from build123d import *

# Parameters (mm, degrees)
F1_DEPTH = 25.4
F2_W     = 25.4
F2_H     = 12.7
F3_DEPTH = 25.4
F4_R     = 6.35
F5_DEPTH = 76.201
F6_R     = 12.7


with BuildPart() as f1:
    # F0 (on Front) → F1 (new body, symmetric)
    with BuildSketch(Plane.XZ):
        Polygon((0, 38.1), (0, 0), (76.2, 0), (76.2, 12.7), (50.8, 12.7), (50.8, 25.4), (25.4, 25.4), (25.4, 50.8), (12.7, 50.8), align=None)
        Polygon((38.1, 50.8), (25.4, 50.8), (25.4, 25.4), (50.8, 25.4), (50.8, 38.1), (38.1, 38.1), align=None)
    extrude(amount=F1_DEPTH, both=True)

    # F2 (on face) → F3 (cut)
    with BuildSketch(Plane.XY.offset(50.8)):
        with Locations((38.1, 19.05)):
            Rectangle(F2_W, F2_H)
        with Locations((38.1, -19.05)):
            Rectangle(F2_W, F2_H)
    extrude(amount=-F3_DEPTH, mode=Mode.SUBTRACT)

    # F4 (on face) → F5 (cut, through all)
    with BuildSketch(Plane.YZ.offset(76.2)):
        with Locations((0, 12.7)):
            Circle(F4_R)
    extrude(amount=-F5_DEPTH, mode=Mode.SUBTRACT)

    # F6
    f6_edges = [f1.edges().sort_by_distance(p)[0] for p in [
        (76.2, -25.4, 6.35),
        (76.2, 25.4, 6.35),
    ]]
    fillet(f6_edges, radius=F6_R)


solid = f1.part
Part model, mm, in its own coordinate system. A direction names the side the tool comes from. Coordinates: 2 decimals unless noted, no trailing zeros. Order: outer loops, then holes, each group sorted by start corner. A loop starts at its lowest first (then second) coordinate and runs counter-clockwise, first axis right, second up.
(1) Tool access for faces 1 (the face through (24, -25.4, 20)), 2 (the face through (38, 0, 0)), 3 (the face through (64, -16, 12.7)), 4 (the face through (38, 19, 25.4)), 5 (the face through (25.4, -19, 38)): list every direction of +Z, -Z, +X, -X, +Y, -Y with a clear straight run to the whole face (end or side of a thin tool).
Check sheet entries:
face 1: +Z, -Z, +X, -X, -Y
face 2: -Z, +X, -X, +Y, -Y
face 3: +Z, +X, +Y, -Y
face 4: +Z, +X, +Y
face 5: +Z, +X, -Y
(2) Probe L1, parallel to X at y = 14, z = 30; L2, parallel to Z at x = 31.5, y = 2; L3, parallel to Z at x = 60, y = 0. List the from-to ranges inside material, lowest first.
Check sheet entries:
L1: x = 0 to 25.4
L2: z = 0 to 6.67, 18.73 to 50.8
L3: z = 0 to 6.35
(3) Pin check, flat tips, straight feed: pin 1 Ø10 at (y, z) = (16.5, 43) entering from +X; pin 2 Ø7.5 at (x, z) = (33.5, 36) entering from -Y; pin 3 Ø14 at (y, z) = (-19, 36.5) entering from +X; pin 4 Ø7.5 at (y, z) = (0, 12.7) entering from +X. Stop position of each tip, or through.
Check sheet entries:
pin 1: stops at x = 38.1
pin 2: stops at y = -12.7
pin 3: stops at x = 50.8
pin 4: passes through
(4) Slice it at B-B, the plane y = 5. Write the cut outline in (x, z).
Check sheet entries:
outline: (0, 0) - (76.2, 0) - (76.2, 8.79) - (0, 8.79) - close; (0, 16.61) - (50.8, 16.61) - (50.8, 38.1) - (38.1, 38.1) - (38.1, 50.8) - (12.7, 50.8) - (0, 38.1) - close
(5) Slice it at D-D, the plane x = 30.5. Write the cut outline in (y, z), and give its area (3 significant figures).
Check sheet entries:
outline: (-25.4, 0) - (25.4, 0) - (25.4, 25.4) - (12.7, 25.4) - (12.7, 50.8) - (-12.7, 50.8) - (-12.7, 25.4) - (-25.4, 25.4) - close; hole circle Ø12.7 at (0, 12.7)
area: 1,810 mm2
(6) Pull direction Y, two halves, no side cores. Call faces 6 (the face through (38, -19, 25.4)), 7 (the face through (72.38, -21.78, 6.44)), 8 (the face through (30.167, 2.93, 7.066)): pulls with the +Y half, pulls with the -Y half, needs draft (parallel to the pull), parting line crosses it, or undercut.
Check sheet entries:
face 6: needs draft
face 7: pulls with the -Y half
face 8: undercut
(7) Slice it at A-A, the plane x = 49. Write the cut outline in (y, z), and give its area (3 significant figures).
Check sheet entries:
outline: (-25.4, 0) - (25.4, 0) - (25.4, 25.4) - (12.7, 25.4) - (12.7, 38.1) - (-12.7, 38.1) - (-12.7, 25.4) - (-25.4, 25.4) - close; hole circle Ø12.7 at (0, 12.7)
area: 1,490 mm2
(8) Slice it at C-C, the plane z = 39. Write the cut outline in (x, y), and give its area (3 significant figures).
Check sheet entries:
outline: (0.9, -25.4) - (25.4, -25.4) - (25.4, -12.7) - (38.1, -12.7) - (38.1, 12.7) - (25.4, 12.7) - (25.4, 25.4) - (0.9, 25.4) - close
area: 1,570 mm2
